The model under review builds one solid part; all positions refer to its coordinate system, in mm. A direction names the side the tool comes from. Round coordinates to 2 decimals unless told otherwise and drop trailing zeros. Order: outer loops, then holes, each group sorted by start corner. A loop starts at its lowest first (then second) coordinate and runs counter-clockwise, first axis right, second up. Notation, with made-up numbers: M -5.75,26.5 L 39.25,26.5 A20 cw 39.25,35.5 Z; hole C -39.75,11 d7. An arc over 180 degrees is marked long. Use a Markdown table: item, result. Add a question column.
1. Consider section B-B on z = 20. State the section outline as (x, y) points.
2. Insertion check: P1, Ø6, axis at x = 13, z = 128.5, coming from the -Y side; P2, Ø6, axis at y = 17, z = 46, coming from the +X side; P3, Ø10, axis at y = 18.5, z = 33, coming from the +X side. Each pin has a flat end and moves straight along its axis. Give the tip position at first contact, or say it passes through.
3. To check wall thickness, follow probe 1 along X at (y, z) = (21.5, 30.5); probe 2 along X at (y, z) = (26.5, 68.5); probe 3 along Y at (x, z) = (-17, 71). State the ranges of each line that lie inside material, in increasing order.
4. Consider section A-A on y = 21.75. State the section outline as (x, z) points, then the cut area to 3 significant figures.
5. The part is to be moulded in two halves that separate along X. For faces 1 (the flat face through (10, 26, 254)), 2 (the flat face through (-46.168, 21, 38)), 3 (the cylindrical face through (-8.46, 28.68, 37.57)), say which applies: +X half, -X half, draft (parallel to the pull), parting line (faces both ways), or undercut.
6. Consider section D-D on x = 12.5. State the section outline as (y, z) points.
7. For faces 4 (the flat face through (-32, 17.527, 38)), 5 (the flat face through (-44, 30.227, 38)), 6 (the cylindrical face through (19.135, 28.2, 125.222)), list the 3-axis set-ups (+Z, -Z, +X, -X, +Y, -Y) from which the entire face can be reached by the end or side of a thin tool; tool diameter is ignored.
8. Consider section C-C on x = -33.5. State the section outline as (y, z) points.
from build123d import *

# Parameters (mm, degrees)
F1_DEPTH = 76.2
F2_R     = 9.333674
F3_DEPTH = 254


with BuildPart() as f1:
    # F0 (on Top) → F1 (new body)
    with BuildSketch(Plane.XY):
        with BuildLine():
            Line((-41.087765, 30.226878), (-46.167765, 30.226878))
            Line((-46.167765, 30.226878), (-46.167765, 12.446878))
            Line((-46.167765, 12.446878), (-16.285702, 12.446878))
            ThreePointArc((-16.285702, 12.446878), (-8.142851, 28.683026), (0, 12.446878))
            Line((0, 12.446878), (5.08, 12.446878))
            ThreePointArc((5.08, 12.446878), (-5.831418, 33.329758), (-23.307765, 17.526878))
            Line((-23.307765, 17.526878), (-41.087765, 17.526878))
            Line((-41.087765, 17.526878), (-41.087765, 30.226878))
        make_face()
    extrude(amount=F1_DEPTH)

    # F2 (on Top) → F3 (join)
    with BuildSketch(Plane.XY):
        with Locations((10.232405, 25.396086)):
            Circle(F2_R)
    extrude(amount=F3_DEPTH)


solid = f1.part
Answer block:
| question | item | result |
|---|---|---|
| 1 | outline | M -46.17,12.45 L -16.29,12.45 A10.16 cw long 0,12.45 L 5.08,12.45 A14.9 ccw 6.34,16.91 A9.33 ccw long 1.82,29.45 A14.9 ccw -23.31,17.53 L -41.09,17.53 L -41.09,30.23 L -46.17,30.23 Z |
| 2 | P1 | y = 16.06 |
| 2 | P2 | x = 17.85 |
| 2 | P3 | x = 19.37 |
| 3 | probe 1 | -46.17 to -41.09, -23.08 to -17.86, 1.57 to 18.71 |
| 3 | probe 2 | -46.17 to -41.09, -21.13 to -14.44, -1.85 to 19.5 |
| 3 | probe 3 | 12.45 to 13.55, 23.5 to 30.87 |
| 4 | outline | M -46.17,0 L -41.09,0 L -41.09,76.2 L -46.17,76.2 Z; M -23.03,0 L -17.78,0 L -17.78,76.2 L -23.03,76.2 Z; M 1.49,0 L 18.82,0 L 18.82,254 L 1.64,254 L 1.64,76.2 L 1.49,76.2 Z |
| 4 | area | 5,160 mm^2 |
| 5 | face 1 | draft |
| 5 | face 2 | -X half |
| 5 | face 3 | undercut |
| 6 | outline | M 16.34,0 L 34.45,0 L 34.45,254 L 16.34,254 Z |
| 7 | face 4 | +Z, -Z, +Y |
| 7 | face 5 | +Z, -Z, -X, +Y |
| 7 | face 6 | +Z |
| 8 | outline | M 12.45,0 L 17.53,0 L 17.53,76.2 L 12.45,76.2 Z |
